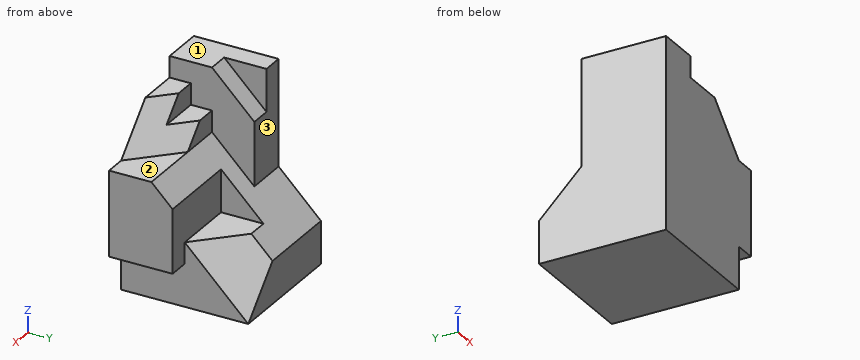
```python
from build123d import *

# Parameters (mm, degrees)
SKETCH1_W           = 7
SKETCH1_H           = 6
BOSS_EXTRUDE1_DEPTH = 9
CUT_EXTRUDE1_DEPTH  = 2
CUT_EXTRUDE2_DEPTH  = 1
CUT_EXTRUDE3_DEPTH  = 6
SKETCH8_W           = 1
SKETCH8_H           = 4
CUT_EXTRUDE6_DEPTH  = 2
CUT_EXTRUDE7_DEPTH  = 1
SKETCH11_W          = 2
SKETCH11_H          = 1
CUT_EXTRUDE9_DEPTH  = 3
CUT_EXTRUDE11_DEPTH = 3
CUT_EXTRUDE12_DEPTH = 1
CUT_EXTRUDE13_DEPTH = 6
CUT_EXTRUDE14_DEPTH = 5
CUT_EXTRUDE16_DEPTH = 5
CUT_EXTRUDE17_DEPTH = 6.773502692
BOSS_EXTRUDE2_DEPTH = 4
CUT_EXTRUDE19_DEPTH = 4
CUT_EXTRUDE20_DEPTH = 3
CUT_EXTRUDE22_DEPTH = 6.773502692
CUT_EXTRUDE23_DEPTH = 10


with BuildPart() as part:
    # Sketch1 → Boss-Extrude1 (new body)
    with BuildSketch(Plane.XY):
        Rectangle(SKETCH1_W, SKETCH1_H)
    extrude(amount=BOSS_EXTRUDE1_DEPTH)

    # Sketch2 → Cut-Extrude1 (cut)
    with BuildSketch(Plane.ZY.offset(3.5)):
        Polygon((2, 3), (4, 1), (9, 1), (9, 3), align=None)
    extrude(amount=-CUT_EXTRUDE1_DEPTH, mode=Mode.SUBTRACT)

    # Sketch3 → Cut-Extrude2 (cut)
    with BuildSketch(Plane(origin=(3.5, 0, 0), x_dir=(0, 0, -1), z_dir=(1, 0, 0))):
        Polygon((0, -3), (-2, -3), (-2, 0), (-3, 0), (0, 3), align=None)
    extrude(amount=-CUT_EXTRUDE2_DEPTH, mode=Mode.SUBTRACT)

    # Sketch5 → Cut-Extrude3 (cut, through all)
    with BuildSketch(Plane.ZY.offset(1.5)):
        Polygon((2, 3), (4, 1), (9, 1), (9, 3), align=None)
    extrude(amount=-CUT_EXTRUDE3_DEPTH, mode=Mode.SUBTRACT)

    # Sketch8 → Cut-Extrude6 (cut)
    with BuildSketch(Plane(origin=(0, 3, 0), x_dir=(1, 0, 0), z_dir=(0, 1, 0))):
        with Locations((3, -2)):
            Rectangle(SKETCH8_W, SKETCH8_H)
    extrude(amount=-CUT_EXTRUDE6_DEPTH, mode=Mode.SUBTRACT)

    # Sketch9 → Cut-Extrude7 (cut)
    with BuildSketch(Plane(origin=(3.5, 0, 0), x_dir=(0, 0, -1), z_dir=(1, 0, 0))):
        Polygon((-2, 1), (-3, 0), (-5, 0), (-5, 1), align=None)
    extrude(amount=-CUT_EXTRUDE7_DEPTH, mode=Mode.SUBTRACT)

    # Sketch11 → Cut-Extrude9 (cut)
    with BuildSketch(Plane(origin=(3.5, 0, 0), x_dir=(0, 0, -1), z_dir=(1, 0, 0))):
        with Locations((-5, 0.5)):
            Rectangle(SKETCH11_W, SKETCH11_H)
    extrude(amount=-CUT_EXTRUDE9_DEPTH, mode=Mode.SUBTRACT)

    # Sketch13 → Cut-Extrude11 (cut)
    with BuildSketch(Plane(origin=(2.5, 0, 0), x_dir=(0, 0, -1), z_dir=(1, 0, 0))):
        Polygon((-5, 0), (-3, 0), (-3, 2), align=None)
    extrude(amount=-CUT_EXTRUDE11_DEPTH, mode=Mode.SUBTRACT)

    # Sketch14 → Cut-Extrude12 (cut)
    with BuildSketch(Plane(origin=(0.5, 0, 0), x_dir=(0, 0, -1), z_dir=(1, 0, 0))):
        Polygon((-4, 1), (-5, 0), (-6, 0), (-6, 1), align=None)
    extrude(amount=-CUT_EXTRUDE12_DEPTH, mode=Mode.SUBTRACT)

    # Sketch15 → Cut-Extrude13 (cut)
    with BuildSketch(Plane(origin=(3.5, 0, 0), x_dir=(0, 0, -1), z_dir=(1, 0, 0))):
        Polygon((-7, 1), (-9, -1), (-9, 1), align=None)
    extrude(amount=-CUT_EXTRUDE13_DEPTH, mode=Mode.SUBTRACT)

    # Sketch17 → Cut-Extrude14 (cut)
    with BuildSketch(Plane(origin=(3.5, 0, 0), x_dir=(0, 0, -1), z_dir=(1, 0, 0))):
        Polygon((-5, 0), (-6, 0), (-6, 1), (-7, 1), (-9, -1), (-9, -3), (-6, -3), (-6, -1), align=None)
    extrude(amount=-CUT_EXTRUDE14_DEPTH, mode=Mode.SUBTRACT)

    # Sketch18 → Cut-Extrude16 (cut)
    with BuildSketch(Plane(origin=(3.5, 0, 0), x_dir=(0, 0, -1), z_dir=(1, 0, 0))):
        Polygon((-3, 2), (-5, 0), (-6, 0), (-6, 1), align=None)
    extrude(amount=-CUT_EXTRUDE16_DEPTH, mode=Mode.SUBTRACT)

    # Sketch20 → Cut-Extrude17 (cut, through all)
    with BuildSketch(Plane(origin=(1.833333333, 1.833333333, 1.833333333), x_dir=(0.816496581, -0.40824829, -0.40824829), z_dir=(0.577350269, 0.577350269, 0.577350269))):
        Polygon((-1.632993162, 0.707106781), (-1.632993162, -0.707106781), (0.816496581, -2.121320344), (0.816496581, 2.121320344), align=None)
    extrude(amount=CUT_EXTRUDE17_DEPTH, mode=Mode.SUBTRACT)

    # Sketch21 → Boss-Extrude2 (add)
    with BuildSketch(Plane(origin=(-1.5, 0, 0), x_dir=(0, 0, -1), z_dir=(1, 0, 0))):
        Polygon((-6, -1), (-7, -1), (-7, -2), (-8, -2), (-8, -3), (-6, -3), align=None)
    extrude(amount=BOSS_EXTRUDE2_DEPTH)

    # Sketch24 → Cut-Extrude19 (cut)
    with BuildSketch(Plane(origin=(1.833333333, 1.833333333, 1.833333333), x_dir=(0.816496581, -0.40824829, -0.40824829), z_dir=(0.577350269, 0.577350269, 0.577350269))):
        Polygon((0.816496581, -6.363961031), (-1.632993162, -4.949747468), (-2.857738033, -5.656854249), (-1.632993162, -7.778174593), align=None)
    extrude(amount=CUT_EXTRUDE19_DEPTH, mode=Mode.SUBTRACT)

    # Sketch25 → Cut-Extrude20 (cut, through all)
    with BuildSketch(Plane(origin=(0, -1, 0), x_dir=(1, 0, 0), z_dir=(0, 1, 0))):
        Polygon((2.5, -6), (0.5, -8), (2.5, -8), align=None)
    extrude(amount=-CUT_EXTRUDE20_DEPTH, mode=Mode.SUBTRACT)

    # Sketch26 → Cut-Extrude22 (cut, through all)
    with BuildSketch(Plane(origin=(1.833333333, 1.833333333, 1.833333333), x_dir=(0.816496581, -0.40824829, -0.40824829), z_dir=(0.577350269, 0.577350269, 0.577350269))):
        Polygon((-1.632993162, -6.363961031), (-2.857738033, -7.071067812), (-1.632993162, -7.778174593), align=None)
    extrude(amount=CUT_EXTRUDE22_DEPTH, mode=Mode.SUBTRACT)

    # Sketch28 → Cut-Extrude23 (cut)
    with BuildSketch(Plane.XY.offset(6)):
        Polygon((0.5, -1), (2.5, -1), (2.5, -3), align=None)
    extrude(amount=CUT_EXTRUDE23_DEPTH, mode=Mode.SUBTRACT)


solid = part.part
```
The model under review builds one solid part; all positions refer to its coordinate system, in mm. Face numbers are marked on the shaded views. A direction names the side the tool comes from. Give positions to 0.01 mm unless a question says otherwise; leave off trailing zeros. Write each loop counter-clockwise with the first axis right and the second up, starting at its lowest first coordinate (ties: lowest second). Pieces come first, ordered by that corner, then holes.
(1) Consider section A-A, the plane x = -2. Give the boundary of the cut face in (y, z), and give its area (3 significant figures).
(2) To check wall thickness, follow L1, parallel to Y at x = 3, z = 5.5; L2, parallel to X at y = -2.5, z = 8.25; L3, parallel to Z at x = -2.5, y = 2. State the ranges of each line that lie inside material, in increasing order.
(3) Consider section C-C, the plane z = 7.25. Give the boundary of the cut face in (x, y), and give its area (3 significant figures).
(4) Tool access review of the marked faces 1, 2 and 3: name each direction out of +Z, -Z, +X, -X, +Y, -Y from which nothing blocks a thin tool from reaching the whole face with its end or side.
(5) For P1, Ø0.9, axis at y = -0.5, z = 1.5, coming from the +X side; P2, Ø2.5, axis at x = 2, z = 3, coming from the +Y side; P3, Ø2, axis at x = -2.5, z = 5.5, coming from the +Y side, all flat-tipped, find the tip position at first contact; note any pin that passes through.
(6) Consider section D-D, the plane y = 0.25. Give the boundary of the cut face in (x, z).
(7) Consider section B-B, the plane y = 1.5. Give the boundary of the cut face in (x, z), and give its area (3 significant figures).
Returned:
1. outline: (-3, 0) - (3, 0) - (3, 2) - (1, 4) - (1, 7) - (-1, 9) - (-3, 9) - close
1. area: 40.0 mm2
2. L1: y = -3 to -0.5
2. L2: x = -3.5 to -1.5
2. L3: z = 0 to 3
3. outline: (-3.5, -3) - (1.25, -3) - (0.25, -2) - (-1.5, -2) - (-1.5, 0.75) - (-2.5, 0.75) - (-2.5, 1) - (-3.5, 1) - close
3. area: 10.0 mm2
4. face 1: +Z, +X, -X, +Y, -Y
4. face 2: +Z, +X, +Y
4. face 3: +Z, +X, -X, +Y
5. P1: stops at x = 2.5
5. P2: stops at y = 2.27
5. P3: stops at y = 1
6. outline: (-3.5, 0) - (2.5, 0) - (2.5, 2.75) - (2.25, 3) - (-0.5, 3) - (-0.5, 4.75) - (-1.5, 4.75) - (-1.5, 7.75) - (-2.5, 7.75) - (-2.5, 9) - (-3.5, 9) - close
7. outline: (-3.5, 0) - (2.5, 0) - (2.5, 1.5) - (1, 3) - (-0.5, 3) - (-0.5, 3.5) - (-3.5, 3.5) - close
7. area: 18.4 mm2
